```python
from build123d import *

# Parameters (mm, degrees)
ESQUISSE1_W             = 40
ESQUISSE1_H             = 4
BOSS_EXTRU_2_DEPTH      = 2
ESQUISSE2_W             = 1
ESQUISSE2_H             = 4
ENL_V_MAT_EXTRU_1_DEPTH = 40
CONG_1_R                = 1
CONG_2_R                = 1


with BuildPart() as part:
    # Esquisse1 → Boss.-Extru.2 (new body)
    with BuildSketch(Plane.XY):
        Rectangle(ESQUISSE1_W, ESQUISSE1_H)
        Polygon((145, 7.5), (145, -7.5), (20, -7.5), (20, -2), (20, 2), (20, 7.5), align=None)
    extrude(amount=BOSS_EXTRU_2_DEPTH)

    # Esquisse2 → Enlèv. mat.-Extru.1 (cut)
    with BuildSketch(Plane.ZY.offset(20)):
        with Locations((1.5, 0)):
            Rectangle(ESQUISSE2_W, ESQUISSE2_H)
    extrude(amount=-ENL_V_MAT_EXTRU_1_DEPTH, mode=Mode.SUBTRACT)

    # Congé1
    cong_1_edges = [part.edges().sort_by_distance(p)[0] for p in [
        (82.5, -7.5, 0),
        (82.5, -7.5, 2),
        (82.5, 7.5, 2),
        (82.5, 7.5, 0),
    ]]
    fillet(cong_1_edges, radius=CONG_1_R - 0.0001)  # a hair under: the kernel refuses the full size

    # Congé2
    cong_2_edges = [part.edges().sort_by_distance(p)[0] for p in [
        (145, 0, 0),
        (145, 0, 2),
        (145, 7.207136071, 0.292863929),
        (145, 7.207136071, 1.707136071),
        (145, -7.207136071, 1.707136071),
        (145, -7.207136071, 0.292863929),
    ]]
    fillet(cong_2_edges, radius=CONG_2_R - 0.0001)  # a hair under: the kernel refuses the full size


solid = part.part
```
Input: part model. Units: mm. Frame: model coordinates. A direction names the side the tool comes from. Coordinates: 2 decimals unless noted, no trailing zeros. Write each loop counter-clockwise with the first axis right and the second up, starting at its lowest first coordinate (ties: lowest second). Pieces come first, ordered by that corner, then holes. Notation, with made-up numbers: (73, -25.75) -> (128, -25.75) arc R31 ccw to (128, 10.25) -> close; hole circle Ø6 at (-21, 41.25). An arc over 180 degrees is marked (long way). Write each question's results on one line, items separated by ' | '.
Item 1: Material intervals for probe 1 along Y at (x, z) = (136, 1.1) (3 decimals); probe 2 along Y at (x, z) = (6.5, 0.15); probe 3 along X at (y, z) = (2.5, 0.85), sorted ascending.
Conclusion:
probe 1: y = -7.495 to 7.495 | probe 2: y = -2 to 2 | probe 3: x = 20 to 144.99
Item 2: Pin query (flat end, axial travel): pin 1 Ø0.5 at (x, z) = (-1, 0.5) entering from -Y; pin 2 Ø4.5 at (x, y) = (9.5, -0.5) entering from +Z. Return the tip coordinate at first contact, or that it passes through.
Conclusion:
pin 1: stops at y = -2 | pin 2: stops at z = 1
Item 3: Section query D-D on x = 4.5. Return loops of the section in (y, z), plus the area to 3 significant figures.
Conclusion:
outline: (-2, 0) -> (2, 0) -> (2, 1) -> (-2, 1) -> close | area: 4.00 mm^2
Item 4: Set-up query: faces 1 (the flat face through (0, 0, 1)), 2 (the flat face through (81, 0, 2)). Return all of +Z, -Z, +X, -X, +Y, -Y with unobstructed straight access to the full face (end or side cutting, diameter ignored); none if empty.
Conclusion:
face 1: +Z, -X, +Y, -Y | face 2: +Z, +X, -X, +Y, -Y
Item 5: Section query C-C on z = 0.45. Return loops of the section in (x, y).
Conclusion:
outline: (-20, -2) -> (20, -2) -> (20, -7.34) -> (144, -7.34) arc R0.84 ccw to (144.84, -6.5) -> (144.84, 6.5) arc R0.84 ccw to (144, 7.34) -> (20, 7.34) -> (20, 2) -> (-20, 2) -> close
